Can you work these out from the model? Positions are in its coordinate system, mm. Coordinates: 2 decimals unless noted, no trailing zeros. Order: outer loops, then holes, each group sorted by start corner. A loop starts at its lowest first (then second) coordinate and runs counter-clockwise, first axis right, second up. Notation, with made-up numbers: M 46.25,-40 L 57.25,-40 A25 ccw 57.25,-25 Z; hole C 29.25,16 d8. An arc over 180 degrees is marked long. Answer as a JSON object with one key per item and string values.
from build123d import *

# Parameters (mm, degrees)
SKETCH_1_W             = 30
SKETCH_1_H             = 31
SM_BASE_FLANGE_1_DEPTH = 1.5
HOLE_WIZARD_M3_1_D     = 3.4
HOLE_WIZARD_M3_1_DEPTH = 20
HOLE_WIZARD_M3_1_TIP   = 1.021463052


# Sheet-metal steps are written as plain solids
with BuildPart() as part:
    # Sketch 1 → 基体-法兰1 (new body)
    with BuildSketch(Plane(origin=(0, 0, 0), x_dir=(0, 0, -1), z_dir=(1, 0, 0))):
        Rectangle(SKETCH_1_W, SKETCH_1_H)
    extrude(amount=-SM_BASE_FLANGE_1_DEPTH)

    # M3 间隙孔1
    with Locations(Plane(origin=(0, 0, 0), x_dir=(0, 0, -1), z_dir=(1, 0, 0))):
        with Locations((-12, 12.5), (12, 12.5), (12, -12.5), (-12, -12.5)):
            Hole(HOLE_WIZARD_M3_1_D / 2, depth=HOLE_WIZARD_M3_1_DEPTH)
            with Locations((0, 0, -(HOLE_WIZARD_M3_1_DEPTH + HOLE_WIZARD_M3_1_TIP / 2))):  # 118° drill point
                Cone(0, HOLE_WIZARD_M3_1_D / 2, HOLE_WIZARD_M3_1_TIP, mode=Mode.SUBTRACT)


solid = part.part
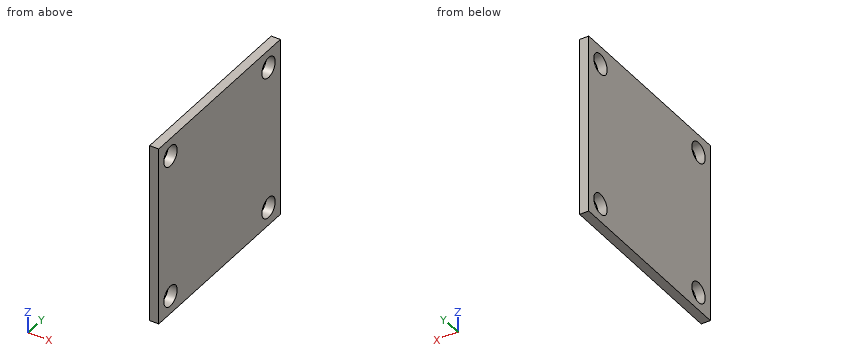
Item 1: Please list where these lines run through material, in increasing order: line 1 (Y direction, x = -0.35, z = 12); line 2 (Y direction, x = -0.6, z = -11); line 3 (Z direction, x = -0.75, y = -11).
Answers follow:
{"line 1": "y = -15.5 to -14.2, -10.8 to 10.8, 14.2 to 15.5", "line 2": "y = -15.5 to -13.87, -11.13 to 11.13, 13.87 to 15.5", "line 3": "z = -15 to -12.8, -11.2 to 11.2, 12.8 to 15"}
Item 2: I want a section at B-B, the plane y = -12.5. Write out the boundary of the cut face in (x, z).
Answers follow:
{"outline": "M -1.5,-15 L 0,-15 L 0,-13.7 L -1.5,-13.7 Z; M -1.5,-10.3 L 0,-10.3 L 0,10.3 L -1.5,10.3 Z; M -1.5,13.7 L 0,13.7 L 0,15 L -1.5,15 Z"}
Item 3: I want a section at A-A, the plane z = 12. Write out the boundary of the cut face in (x, y).
Answers follow:
{"outline": "M -1.5,-15.5 L 0,-15.5 L 0,-14.2 L -1.5,-14.2 Z; M -1.5,-10.8 L 0,-10.8 L 0,10.8 L -1.5,10.8 Z; M -1.5,14.2 L 0,14.2 L 0,15.5 L -1.5,15.5 Z"}
Item 4: I want a section at C-C, the plane x = -1. Write out the boundary of the cut face in (y, z).
Answers follow:
{"outline": "M -15.5,-15 L 15.5,-15 L 15.5,15 L -15.5,15 Z; hole C -12.5,-12 d3.4; hole C -12.5,12 d3.4; hole C 12.5,-12 d3.4; hole C 12.5,12 d3.4"}
